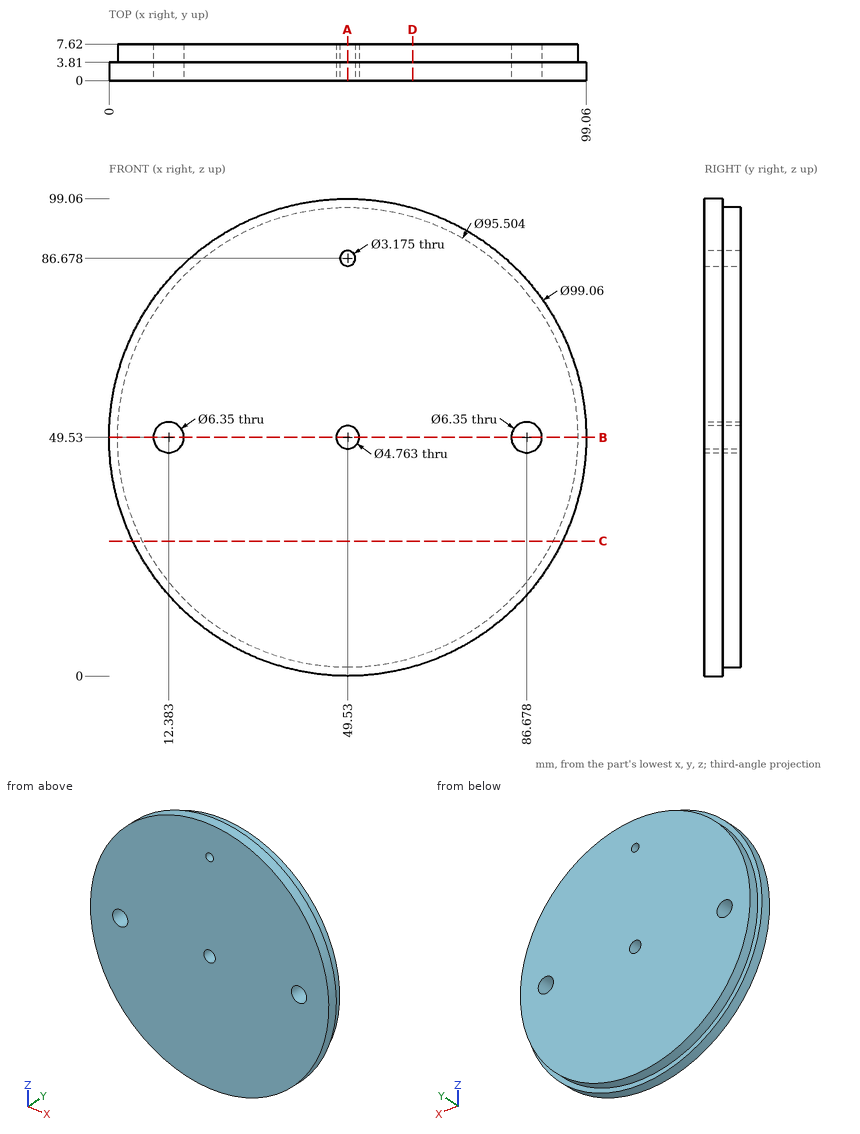
Drawing for the job (mm, zero at the part's lowest x, y, z). Round coordinates to 2 decimals unless told otherwise and drop trailing zeros. Loops run counter-clockwise (first coordinate to the right, second up) from the corner with the lowest first, then second, coordinate; pieces in that order, holes last. Notation, with made-up numbers: (-18.75, 48) - (29.25, 48) arc R10 ccw to (29.25, 53) - close; hole circle Ø10 at (89, 47.5). An arc over 180 degrees is marked (long way). Write each question's results on one line, items separated by ' | '.
(1) Saw through at D-D, the plane x = 63. List the corners of the cut face in (y, z), then the cut area to 3 significant figures.
Answer below:
outline: (0, 1.87) - (3.81, 1.87) - (3.81, 3.72) - (7.62, 3.72) - (7.62, 95.34) - (3.81, 95.34) - (3.81, 97.19) - (0, 97.19) - close | area: 712 mm^2
(2) Wall check: L1, parallel to X at y = 1.5, z = 49.53; L2, parallel to X at y = 3.25, z = 52 (1 decimal); L3, parallel to Z at x = 88, y = 1 (1 decimal). Give the ranges that are in metal, low to high.
Answer below:
L1: x = 0 to 9.21, 15.56 to 47.15, 51.91 to 83.5, 89.85 to 99.06 | L2: x = 0.1 to 10.4, 14.4 to 84.7, 88.7 to 99 | L3: z = 18.3 to 46.6, 52.4 to 80.7
(3) Saw through at B-B, the plane z = 49.53. List the corners of the cut face in (x, y), then the cut area to 3 significant figures.
Answer below:
outline: (0, 0) - (9.21, 0) - (9.21, 7.62) - (1.78, 7.62) - (1.78, 3.81) - (0, 3.81) - close; (15.56, 0) - (47.15, 0) - (47.15, 7.62) - (15.56, 7.62) - close; (51.91, 0) - (83.5, 0) - (83.5, 7.62) - (51.91, 7.62) - close; (89.85, 0) - (99.06, 0) - (99.06, 3.81) - (97.28, 3.81) - (97.28, 7.62) - (89.85, 7.62) - close | area: 608 mm^2
(4) Pin check, flat tips, straight feed: pin 1 (4 mm diameter, centred on x = 49.53, z = 49.53, fed in from +Y); pin 2 (1.5 mm diameter, centred on y = 5, z = 47, fed in from +X); pin 3 (8.5 mm diameter, centred on x = 12.38, z = 49.53, fed in from +Y); pin 4 (2 mm diameter, centred on x = 37, y = 3.5, fed in from -Z). Stop position of each tip, or through.
Answer below:
pin 1: passes through | pin 2: stops at x = 97.25 | pin 3: stops at y = 7.62 | pin 4: stops at z = 1.36
(5) Saw through at C-C, the plane z = 28. List the corners of the cut face in (x, y) (1 decimal).
Answer below:
outline: (4.9, 0) - (94.1, 0) - (94.1, 3.8) - (92.2, 3.8) - (92.2, 7.6) - (6.9, 7.6) - (6.9, 3.8) - (4.9, 3.8) - close
(6) Saw through at A-A, the plane x = 49.53. List the corners of the cut face in (y, z) (1 decimal), then the cut area to 3 significant figures.
Answer below:
outline: (0, 0) - (3.8, 0) - (3.8, 1.8) - (7.6, 1.8) - (7.6, 47.1) - (0, 47.1) - close; (0, 51.9) - (7.6, 51.9) - (7.6, 85.1) - (0, 85.1) - close; (0, 88.3) - (7.6, 88.3) - (7.6, 97.3) - (3.8, 97.3) - (3.8, 99.1) - (0, 99.1) - close | area: 681 mm^2
